```python
from build123d import *

# Parameters (mm, degrees)
BOSS_EXTRUDE1_DEPTH      = 12.7
BOSS_EXTRUDE1_DEPTH_BACK = 12.7
SKETCH2_R                = 4.7625
CUT_EXTRUDE1_DEPTH       = 12.7
SKETCH4_R                = 2.1
CUT_EXTRUDE2_DEPTH       = 3.54


with BuildPart() as part:
    # Sketch1 → Boss-Extrude1 (new body, two sides)
    with BuildSketch(Plane(origin=(0, 0, 0), x_dir=(0, 0, -1), z_dir=(1, 0, 0))) as boss_extrude1_sk:
        Polygon((-25.4, 0), (0, 0), (0, 63.5), (-2.54, 63.5), (-2.54, 2.54), (-25.4, 2.54), align=None)
    extrude(amount=BOSS_EXTRUDE1_DEPTH)
    extrude(boss_extrude1_sk.sketch, amount=-BOSS_EXTRUDE1_DEPTH_BACK)

    # Sketch2 → Cut-Extrude1 (cut)
    with BuildSketch(Plane.XY.offset(2.54)):
        with Locations((0, 50.8)):
            Circle(SKETCH2_R)
    extrude(amount=-CUT_EXTRUDE1_DEPTH, mode=Mode.SUBTRACT)

    # Sketch4 → Cut-Extrude2 (cut, through all)
    with BuildSketch(Plane(origin=(0, 2.54, 0), x_dir=(1, 0, 0), z_dir=(0, 1, 0))):
        with Locations((6.35, -8.255)):
            Circle(SKETCH4_R)
        with Locations((-6.35, -19.685)):
            Circle(SKETCH4_R)
    extrude(amount=-CUT_EXTRUDE2_DEPTH, mode=Mode.SUBTRACT)


solid = part.part
```
Check sheet for the modelled part. Datum: model origin and axes. Units: mm. A direction names the side the tool comes from. Round coordinates to 2 decimals unless told otherwise and drop trailing zeros. Order: outer loops, then holes, each group sorted by start corner. A loop starts at its lowest first (then second) coordinate and runs counter-clockwise, first axis right, second up.
1) Go/stop test with flat-tipped pins: pin 1 Ø4 at (x, z) = (-0.5, 22) entering from -Y; pin 2 Ø5.5 at (x, y) = (0, 50.8) entering from -Z; pin 3 Ø4 at (x, y) = (2.5, 35) entering from +Z; pin 4 Ø6.5 at (x, z) = (6.35, 8.255) entering from +Y. Record where each tip stops, or that it passes through.
2) Tool access check on faces 4 (the flat face through (0, 33, 2.54)), 5 (the cylindrical face through (7.5, 1.3, 6.5)). Record the directions out of +Z, -Z, +X, -X, +Y, -Y that give a thin tool (end or side, any length) a straight path to the whole face; none if there is none.
3) Mould release check, pull along X, two halves, no side actions. Record for faces 1 (the flat face through (-12.7, 22, 2)), 2 (the cylindrical face through (-6.805, 1.288, 21.735)), 3 (the flat face through (0, 63.5, 1)): +X half, -X half, draft (parallel to the pull), parting line (faces both ways), or undercut.
4) Section check B-B (x = 0). Record the boundary of the cut face in (y, z).
5) Section check C-C (x = -9.25). Record the boundary of the cut face in (y, z).
6) Scan lines: line 1 (Y direction, x = 0, z = 1.9); line 2 (Z direction, x = -6.35, y = 1.7) (3 decimals); line 3 (Y direction, x = -6.25, z = 17.5). Record each from-to range of solid material in increasing order.
7) Section check A-A (y = 50.8). Record the boundary of the cut face in (x, z).
8) Section check D-D (z = 21). Record the boundary of the cut face in (x, y).
Result:
1. pin 1: stops at y = 0
1. pin 2: passes through
1. pin 3: stops at z = 2.54
1. pin 4: stops at y = 2.54
2. face 4: +Z, +X, -X, +Y
2. face 5: +Y, -Y
3. face 1: -X half
3. face 2: undercut
3. face 3: draft
4. outline: (0, 0) - (46.04, 0) - (46.04, 2.54) - (2.54, 2.54) - (2.54, 25.4) - (0, 25.4) - close; (55.56, 0) - (63.5, 0) - (63.5, 2.54) - (55.56, 2.54) - close
5. outline: (0, 0) - (63.5, 0) - (63.5, 2.54) - (2.54, 2.54) - (2.54, 25.4) - (0, 25.4) - close
6. line 1: y = 0 to 46.04, 55.56 to 63.5
6. line 2: z = 0 to 17.585, 21.785 to 25.4
6. line 3: y = 0 to 2.54
7. outline: (-12.7, 0) - (-4.76, 0) - (-4.76, 2.54) - (-12.7, 2.54) - close; (4.76, 0) - (12.7, 0) - (12.7, 2.54) - (4.76, 2.54) - close
8. outline: (-12.7, 0) - (-7.99, 0) - (-7.99, 2.54) - (-12.7, 2.54) - close; (-4.71, 0) - (12.7, 0) - (12.7, 2.54) - (-4.71, 2.54) - close
